from build123d import *

# Parameters (mm, degrees)
SKETCH1_W           = 120
SKETCH1_H           = 140
BOSS_EXTRUDE1_DEPTH = 4
SKETCH2_W           = 12
SKETCH2_H           = 23
SKETCH2_H_2         = 34
SKETCH2_R           = 1.1
SKETCH2_R_2         = 2
CUT_EXTRUDE1_DEPTH  = 93.28217596
SKETCH3_W           = 2.5
SKETCH3_H           = 140
BOSS_EXTRUDE2_DEPTH = 4
SKETCH7_W           = 2.5
SKETCH7_H           = 10
BOSS_EXTRUDE6_DEPTH = 12
SKETCH8_W           = 17
SKETCH8_H           = 10
BOSS_EXTRUDE7_DEPTH = 2
SKETCH9_R           = 3.4
BOSS_EXTRUDE8_DEPTH = 2
SKETCH10_W          = 2.5
SKETCH10_H          = 34
CUT_EXTRUDE2_DEPTH  = 96.949205312
FILLET1_R           = 10
FILLET2_R           = 10
FILLET3_R           = 10
FILLET4_R           = 10
FILLET5_R           = 3
FILLET6_R           = 3
FILLET7_R           = 3
FILLET8_R           = 3
SKETCH11_W          = 56
SKETCH11_H          = 90
CUT_EXTRUDE3_DEPTH  = 96.949205312


with BuildPart() as part:
    # Sketch1 → Boss-Extrude1 (new body)
    with BuildSketch(Plane(origin=(0, 0, 0), x_dir=(1, 0, 0), z_dir=(0, 1, 0))):
        Rectangle(SKETCH1_W, SKETCH1_H)
    extrude(amount=BOSS_EXTRUDE1_DEPTH)

    # Sketch2 → Cut-Extrude1 (cut, through all)
    with BuildSketch(Plane(origin=(0, 4, 0), x_dir=(1, 0, 0), z_dir=(0, 1, 0))):
        with Locations((54, 38.5)):
            Rectangle(SKETCH2_W, SKETCH2_H)
        with Locations((-54, 38.5)):
            Rectangle(SKETCH2_W, SKETCH2_H)
        with Locations((54, -38.5)):
            Rectangle(SKETCH2_W, SKETCH2_H)
        with Locations((-54, -38.5)):
            Rectangle(SKETCH2_W, SKETCH2_H)
        with Locations((-54, 0)):
            Rectangle(SKETCH2_W, SKETCH2_H_2)
        with Locations((54, 0)):
            Rectangle(SKETCH2_W, SKETCH2_H_2)
        with Locations(Location((-54, 52.65, 0), (0, 0, 270))):
            Circle(SKETCH2_R)
        with Locations(Location((-54, 24.35, 0), (0, 0, 270))):
            Circle(SKETCH2_R)
        with Locations(Location((-54, -24.35, 0), (0, 0, 270))):
            Circle(SKETCH2_R)
        with Locations(Location((-54, -52.65, 0), (0, 0, 270))):
            Circle(SKETCH2_R)
        with Locations(Location((54, 52.65, 0), (0, 0, 270))):
            Circle(SKETCH2_R)
        with Locations(Location((54, 24.35, 0), (0, 0, 270))):
            Circle(SKETCH2_R)
        with Locations(Location((54, -24.35, 0), (0, 0, 270))):
            Circle(SKETCH2_R)
        with Locations(Location((54, -52.65, 0), (0, 0, 270))):
            Circle(SKETCH2_R)
        with Locations(Location((-54.5, 62, 0), (0, 0, 270))):
            Circle(SKETCH2_R_2)
        with Locations(Location((54.5, 62, 0), (0, 0, 270))):
            Circle(SKETCH2_R_2)
        with Locations(Location((54.5, -62, 0), (0, 0, 270))):
            Circle(SKETCH2_R_2)
        with Locations(Location((-54.5, -62, 0), (0, 0, 270))):
            Circle(SKETCH2_R_2)
    extrude(amount=-CUT_EXTRUDE1_DEPTH, mode=Mode.SUBTRACT)

    # Sketch3 → Boss-Extrude2 (add)
    with BuildSketch(Plane(origin=(0, 4, 0), x_dir=(1, 0, 0), z_dir=(0, 1, 0))):
        with Locations((61.25, 0)):
            Rectangle(SKETCH3_W, SKETCH3_H)
        with Locations((-61.25, 0)):
            Rectangle(SKETCH3_W, SKETCH3_H)
    extrude(amount=-BOSS_EXTRUDE2_DEPTH)

    # Sketch7 → Boss-Extrude6 (add)
    with BuildSketch(Plane.XZ):
        with Locations((46.75, 43.5)):
            Rectangle(SKETCH7_W, SKETCH7_H)
        with Locations((61.25, 43.5)):
            Rectangle(SKETCH7_W, SKETCH7_H)
        with Locations((-61.25, 43.5)):
            Rectangle(SKETCH7_W, SKETCH7_H)
        with Locations((-46.75, 43.5)):
            Rectangle(SKETCH7_W, SKETCH7_H)
        with Locations((-61.25, -43.5)):
            Rectangle(SKETCH7_W, SKETCH7_H)
        with Locations((-46.75, -43.5)):
            Rectangle(SKETCH7_W, SKETCH7_H)
        with Locations((46.75, -43.5)):
            Rectangle(SKETCH7_W, SKETCH7_H)
        with Locations((61.25, -43.5)):
            Rectangle(SKETCH7_W, SKETCH7_H)
    extrude(amount=BOSS_EXTRUDE6_DEPTH)

    # Sketch8 → Boss-Extrude7 (add)
    with BuildSketch(Plane.XZ.offset(12)):
        with Locations((-54, 43.5)):
            Rectangle(SKETCH8_W, SKETCH8_H)
        with Locations((-54, -43.5)):
            Rectangle(SKETCH8_W, SKETCH8_H)
        with Locations((54, -43.5)):
            Rectangle(SKETCH8_W, SKETCH8_H)
        with Locations((54, 43.5)):
            Rectangle(SKETCH8_W, SKETCH8_H)
    extrude(amount=BOSS_EXTRUDE7_DEPTH)

    # Sketch9 → Boss-Extrude8 (add)
    with BuildSketch(Plane.XZ.offset(14)):
        with Locations(Location((54, 43.5, 0), (0, 0, 270))):
            Circle(SKETCH9_R)
        with Locations(Location((-54, 43.5, 0), (0, 0, 270))):
            Circle(SKETCH9_R)
        with Locations(Location((-54, -43.5, 0), (0, 0, 270))):
            Circle(SKETCH9_R)
        with Locations(Location((54, -43.5, 0), (0, 0, 270))):
            Circle(SKETCH9_R)
    extrude(amount=BOSS_EXTRUDE8_DEPTH)

    # Sketch10 → Cut-Extrude2 (cut, through all)
    with BuildSketch(Plane(origin=(0, 4, 0), x_dir=(1, 0, 0), z_dir=(0, 1, 0))):
        with Locations((61.25, 0)):
            Rectangle(SKETCH10_W, SKETCH10_H)
        with Locations((-61.25, 0)):
            Rectangle(SKETCH10_W, SKETCH10_H)
    extrude(amount=-CUT_EXTRUDE2_DEPTH, mode=Mode.SUBTRACT)

    # Fillet1
    fillet1_edges = [part.edges().sort_by_distance(p)[0] for p in [
        (62.5, 2, -70),
    ]]
    fillet(fillet1_edges, radius=FILLET1_R)

    # Fillet2
    fillet2_edges = [part.edges().sort_by_distance(p)[0] for p in [
        (-62.5, 2, -70),
    ]]
    fillet(fillet2_edges, radius=FILLET2_R)

    # Fillet3
    fillet3_edges = [part.edges().sort_by_distance(p)[0] for p in [
        (-62.5, 2, 70),
    ]]
    fillet(fillet3_edges, radius=FILLET3_R)

    # Fillet4
    fillet4_edges = [part.edges().sort_by_distance(p)[0] for p in [
        (62.5, 2, 70),
    ]]
    fillet(fillet4_edges, radius=FILLET4_R)

    # Fillet5
    fillet5_edges = [part.edges().sort_by_distance(p)[0] for p in [
        (62.5, 2, -17),
    ]]
    fillet(fillet5_edges, radius=FILLET5_R)

    # Fillet6
    fillet6_edges = [part.edges().sort_by_distance(p)[0] for p in [
        (-62.5, 2, 17),
    ]]
    fillet(fillet6_edges, radius=FILLET6_R)

    # Fillet7
    fillet7_edges = [part.edges().sort_by_distance(p)[0] for p in [
        (62.5, 2, 17),
    ]]
    fillet(fillet7_edges, radius=FILLET7_R)

    # Fillet8
    fillet8_edges = [part.edges().sort_by_distance(p)[0] for p in [
        (-62.5, 2, -17),
    ]]
    fillet(fillet8_edges, radius=FILLET8_R)

    # Sketch11 → Cut-Extrude3 (cut, through all)
    with BuildSketch(Plane(origin=(0, 4, 0), x_dir=(1, 0, 0), z_dir=(0, 1, 0))):
        Rectangle(SKETCH11_W, SKETCH11_H)
    extrude(amount=-CUT_EXTRUDE3_DEPTH, mode=Mode.SUBTRACT)


solid = part.part
For this review, take the finished solid that the model builds, in its own axes (mm). A direction names the side the tool comes from. Give positions to 0.01 mm unless a question says otherwise; leave off trailing zeros. Loops run counter-clockwise (first coordinate to the right, second up) from the corner with the lowest first, then second, coordinate; pieces in that order, holes last.
Item 1: Take a section at C-C, the plane z = -15. State the section outline as (x, y) points.
Item 2: Insertion check: pin 1 (4.5 mm diameter, centred on y = 1, z = 1.5, fed in from +X); pin 2 (4.5 mm diameter, centred on x = -53, y = 2.5, fed in from +Z); pin 3 (5 mm diameter, centred on x = 53, z = 45, fed in from +Y); pin 4 (4.5 mm diameter, centred on y = 1.5, z = 13, fed in from -X). Each pin has a flat end and moves straight along its axis. Give the tip position at first contact, or say it passes through.
Item 3: Take a section at D-D, the plane x = 36. State the section outline as (y, z) points.
Item 4: Draft analysis for pull direction X (two halves, no side actions). For faces 6 (the flat face through (-48, 2, 0)), 7 (the flat face through (45.5, -7, -44)), 8 (the flat face through (-54, 2, 17)), 9 (the flat face through (-60, -2, 41)), state which applies: +X half, -X half, draft (parallel to the pull), parting line (faces both ways), or undercut.
Item 5: Tool access review of faces 1 (the flat face through (54, -12, -43)), 2 (the flat face through (60, -2, -41)), 3 (the flat face through (-54, -12.2, 48.5)), 4 (the flat face through (-54, -12.2, -38.5)), 5 (the flat face through (54, 2, 50)): name each direction out of +Z, -Z, +X, -X, +Y, -Y from which nothing blocks a thin tool from reaching the whole face with its end or side.
Item 6: For line 1 along X through (y, z) = (2.15, -52.65); line 2 along X through (y, z) = (-5.75, 42); line 3 along X through (y, z) = (1.45, -24.35), list the stretches that pass through material, from the lowest coordinate up.
Item 7: Take a section at A-A, the plane y = -8. Give the number of separate pieces and of enclosed holes in the cut face, and give its area (3 significant figures).
Item 8: Take a section at B-B, the plane x = 0. State the section outline as (y, z) points.
Calculated:
1. outline: (-48, 0) - (-28, 0) - (-28, 4) - (-48, 4) - close; (28, 0) - (48, 0) - (48, 4) - (28, 4) - close
2. pin 1: stops at x = 48
2. pin 2: stops at z = 70
2. pin 3: stops at y = -12
2. pin 4: stops at x = -48
3. outline: (0, -70) - (4, -70) - (4, 70) - (0, 70) - close
4. face 6: -X half
4. face 7: undercut
4. face 8: draft
4. face 9: undercut
5. face 1: +Z, -Z, +Y
5. face 2: +Y
5. face 3: +Z, +X, -X, -Y
5. face 4: +X, -X, -Y
5. face 5: +Y, -Y
6. line 1: x = -62.5 to -55.1, -52.9 to 52.9, 55.1 to 62.5
6. line 2: x = -62.5 to -60, -48 to -45.5, 45.5 to 48, 60 to 62.5
6. line 3: x = -62.5 to -55.1, -52.9 to -28, 28 to 52.9, 55.1 to 62.5
7. separate pieces: 8
7. enclosed holes: 0
7. area: 200 mm2
8. outline: (0, -70) - (4, -70) - (4, -45) - (0, -45) - close; (0, 45) - (4, 45) - (4, 70) - (0, 70) - close
